```python
from build123d import *

# Parameters (mm, degrees)
SKETCH2_R           = 5
BOSS_EXTRUDE1_DEPTH = 2.4892
SKETCH3_R           = 3.175
CUT_EXTRUDE1_DEPTH  = 5.9784
SKETCH4_R           = 4.125
SKETCH4_R_2         = 3.5
CUT_EXTRUDE2_DEPTH  = 0.2
CHAMFER1_SIZE       = 0.1
FILLET1_R           = 0.25


with BuildPart() as part:
    # Sketch2 → Boss-Extrude1 (new body, symmetric)
    with BuildSketch(Plane(origin=(0, 0, 0), x_dir=(0, 0, -1), z_dir=(1, 0, 0))):
        Circle(SKETCH2_R)
    extrude(amount=BOSS_EXTRUDE1_DEPTH, both=True)

    # Sketch3 → Cut-Extrude1 (cut, through all)
    with BuildSketch(Plane(origin=(2.4892, 0, 0), x_dir=(0, 0, -1), z_dir=(1, 0, 0))):
        Circle(SKETCH3_R)
    extrude(amount=-CUT_EXTRUDE1_DEPTH, mode=Mode.SUBTRACT)

    # Sketch4 → Cut-Extrude2 (cut)
    with BuildSketch(Plane(origin=(2.4892, 0, 0), x_dir=(0, 0, -1), z_dir=(1, 0, 0))):
        Circle(SKETCH4_R)
        Circle(SKETCH4_R_2, mode=Mode.SUBTRACT)
    cut_extrude2 = extrude(amount=-CUT_EXTRUDE2_DEPTH, mode=Mode.SUBTRACT)

    # Mirror1: Cut-Extrude2 across plane
    add(cut_extrude2.mirror(Plane(origin=(0, 0, 0), x_dir=(0, 0, 1), z_dir=(1, 0, 0))), mode=Mode.SUBTRACT)

    # Chamfer1
    chamfer1_edges = [part.edges().sort_by_distance(p)[0] for p in [
        (2.4892, 0, 4.125),
        (-2.4892, 0, 5),
        (-2.4892, 0, 3.175),
        (2.4892, 0, 3.175),
    ]]
    chamfer(chamfer1_edges, length=CHAMFER1_SIZE)

    # Fillet1
    fillet1_edges = [part.edges().sort_by_distance(p)[0] for p in [
        (-2.3892, 0, 5),
        (2.4892, 0, 5),
    ]]
    fillet(fillet1_edges, radius=FILLET1_R)


solid = part.part
```
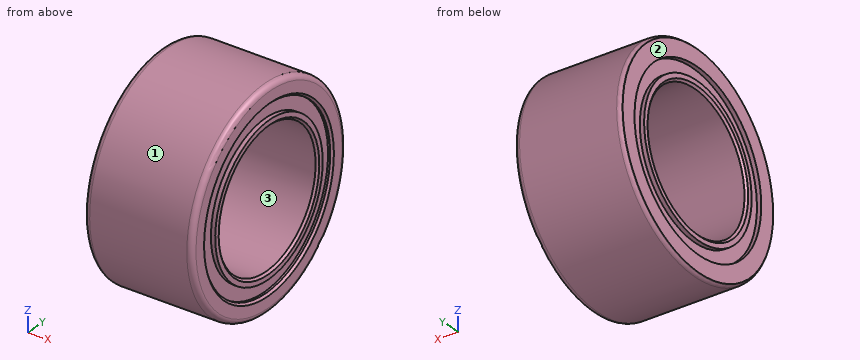
Work out the finished part from the listing and answer in its coordinate system (mm). Face numbers are marked on the shaded views. Coordinates: 2 decimals unless noted, no trailing zeros. Loops run counter-clockwise (first coordinate to the right, second up) from the corner with the lowest first, then second, coordinate; pieces in that order, holes last.
1) Consider probe 1 along Y at (x, z) = (-2.25, 0) (3 decimals); probe 2 along Y at (x, z) = (-0.05, 1.5); probe 3 along Z at (x, y) = (1.35, -1). Determine where each line is inside the solid, lowest interval first.
Results:
probe 1: y = -5 to -3.175, 3.175 to 5
probe 2: y = -4.77 to -2.8, 2.8 to 4.77
probe 3: z = -4.9 to -3.01, 3.01 to 4.9
2) For a pull along Z with two mould halves and no side action, classify the marked faces 1, 2 and 3 as +Z half, -Z half, draft (parallel to the pull), parting line (faces both ways), or undercut.
Results:
face 1: parting line
face 2: draft
face 3: undercut
3) Section A-A (x = -1.5) is taken. Give the vertices of the cut face in (y, z) (3 decimals).
Results:
outline: circle Ø10 at (0, 0); hole circle Ø6.35 at (0, 0)
4) A flat-ended cylindrical pin translates along its axis: pin 1 (1.5 mm diameter, centred on x = 2, z = 2, fed in from +Y). Find the tip coordinate at first contact, or state that the pin passes through.
Results:
pin 1: stops at y = 4.84
